```python
from build123d import *

# Parameters (mm, degrees)
SKETCH1_W           = 12
SKETCH1_H           = 5
BOSS_EXTRUDE1_DEPTH = 5
SKETCH2_R           = 1.5
CUT_EXTRUDE1_DEPTH  = 15.335059136
SKETCH3_R           = 1.5
CUT_EXTRUDE2_DEPTH  = 14.87695255
MOVE_FACE1_BY       = 0.2
MOVE_FACE1_2_BY     = 0.2


with BuildPart() as part:
    # Sketch1 → Boss-Extrude1 (new body)
    with BuildSketch(Plane.XY):
        with Locations((-6.469720142, -0.975038364)):
            Rectangle(SKETCH1_W, SKETCH1_H)
    extrude(amount=BOSS_EXTRUDE1_DEPTH)

    # Sketch2 → Cut-Extrude1 (cut, through all)
    with BuildSketch(Plane.XZ.offset(3.475038364)):
        with Locations(Location((-6.469720142, 2.5, 0), (0, 0, 270))):
            Circle(SKETCH2_R)
    extrude(amount=-CUT_EXTRUDE1_DEPTH, mode=Mode.SUBTRACT)

    # Sketch3 → Cut-Extrude2 (cut, through all)
    with BuildSketch(Plane(origin=(0, 0, 0), x_dir=(-1, 0, 0), z_dir=(0, 0, -1))):
        with Locations((10.469720142, -0.98443785)):
            Circle(SKETCH3_R)
        with Locations(Location((2.469720142, -0.98443785, 0), (0, 0, 180))):
            Circle(SKETCH3_R)
    extrude(amount=-CUT_EXTRUDE2_DEPTH, mode=Mode.SUBTRACT)

    # Move Face1: a face moved inward by 0.2
    extrude(part.faces().sort_by_distance((-0.469720142, -0.975038364, 2.5))[0], amount=MOVE_FACE1_BY, dir=(-1, 0, 0), mode=Mode.SUBTRACT)

    # Move Face1 2: a face moved inward by 0.2
    extrude(part.faces().sort_by_distance((-12.469720142, -0.975038364, 2.5))[0], amount=MOVE_FACE1_2_BY, dir=(1, 0, 0), mode=Mode.SUBTRACT)


solid = part.part
```
CAD build for the part. Positions are in the model's coordinates, mm. Coordinates: 2 decimals unless noted, no trailing zeros. Order: outer loops, then holes, each group sorted by start corner. A loop starts at its lowest first (then second) coordinate and runs counter-clockwise, first axis right, second up.
(1) Mould opens along X. For faces 1 (the face through (-1.039, -1.435, 2.465)), 2 (the face through (-0.67, -1, 2)), 3 (the face through (-7, -1, 0)) say: released by +X, released by -X, zero draft, split by the parting line, or undercut.
Solution:
face 1: undercut
face 2: released by +X
face 3: zero draft
(2) Saw through at B-B, the plane y = -1.75. Write the cut outline in (x, z).
Solution:
outline: (-12.27, 0) - (-11.76, 0) - (-11.76, 5) - (-12.27, 5) - close; (-9.18, 0) - (-3.76, 0) - (-3.76, 5) - (-9.18, 5) - close; (-1.18, 0) - (-0.67, 0) - (-0.67, 5) - (-1.18, 5) - close; hole circle Ø3 at (-6.47, 2.5)
(3) Saw through at A-A, the plane z = 3.5. Write the cut outline in (x, y).
Solution:
outline: (-12.27, -3.48) - (-7.59, -3.48) - (-7.59, 1.52) - (-12.27, 1.52) - close; (-5.35, -3.48) - (-0.67, -3.48) - (-0.67, 1.52) - (-5.35, 1.52) - close; hole circle Ø3 at (-10.47, -0.98); hole circle Ø3 at (-2.47, -0.98)
(4) Drill centre lines: L1, parallel to X at y = -1.8, z = 3.5; L2, parallel to X at y = -1.9, z = 1.15; L3, parallel to Y at x = -3.5, z = 3.6. Where is each one in solid material? Low to high.
Solution:
L1: x = -12.27 to -11.73, -9.21 to -7.59, -5.35 to -3.73, -1.21 to -0.67
L2: x = -12.27 to -11.66, -9.28 to -7.12, -5.82 to -3.66, -1.28 to -0.67
L3: y = -3.48 to -2.07, 0.11 to 1.52
(5) Saw through at C-C, the plane x = -10. Write the cut outline in (y, z).
Solution:
outline: (-3.48, 0) - (-2.41, 0) - (-2.41, 5) - (-3.48, 5) - close; (0.44, 0) - (1.52, 0) - (1.52, 5) - (0.44, 5) - close
(6) Saw through at D-D, the plane y = -1.2. Write the cut outline in (x, z), and give its area (3 significant figures).
Solution:
outline: (-12.27, 0) - (-11.95, 0) - (-11.95, 5) - (-12.27, 5) - close; (-8.99, 0) - (-3.95, 0) - (-3.95, 5) - (-8.99, 5) - close; (-0.99, 0) - (-0.67, 0) - (-0.67, 5) - (-0.99, 5) - close; hole circle Ø3 at (-6.47, 2.5)
area: 21.2 mm2
